Can you work these out from the model? Positions are in its coordinate system, mm. Face numbers are marked on the shaded views. A direction names the side the tool comes from. Give positions to 0.01 mm unless a question says otherwise; leave off trailing zeros. Write each loop counter-clockwise with the first axis right and the second up, starting at its lowest first coordinate (ties: lowest second). Pieces come first, ordered by that corner, then holes. Notation, with made-up numbers: (-34, -29.75) -> (-20, -29.75) arc R14 cw to (-20, -6.75) -> close; hole circle Ø7 at (64, 74). An arc over 180 degrees is marked (long way). One line per item, written item: value.
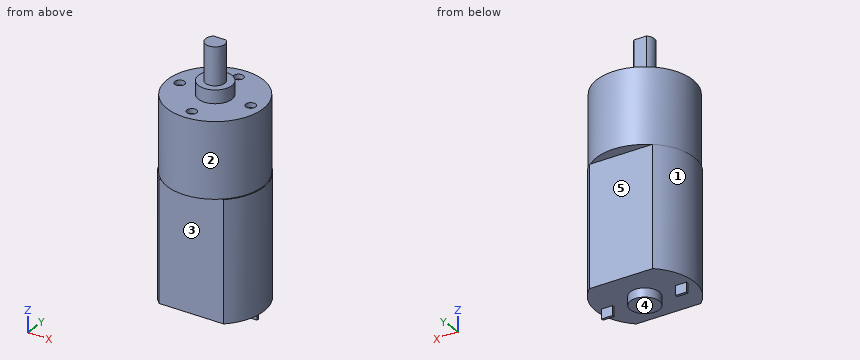
from build123d import *

# Parameters (mm, degrees)
SKETCH1_R                    = 10
GEARBOX_DEPTH                = 15.7
MOTOR_DEPTH                  = 25.1
SKETCH4_R                    = 3.5
OUTPUT_SHAFT_COLLAR_DEPTH    = 2.78
OUTPUT_SHAFT_DEPTH           = 7.87
SKETCH6_R                    = 3.02
BOSS_EXTRUDE11_DEPTH         = 1.86
SKETCH10_W                   = 2.36
SKETCH10_H                   = 0.5
BOSS_EXTRUDE13_DEPTH         = 2
M2_5X0_45_TAPPED_HOLE1_D     = 2.05
M2_5X0_45_TAPPED_HOLE1_DEPTH = 1
M2_5X0_45_TAPPED_HOLE1_TIP   = 0.615882135


with BuildPart() as part:
    # Sketch1 → GearBox (new body)
    with BuildSketch(Plane.XY):
        Circle(SKETCH1_R)
    extrude(amount=GEARBOX_DEPTH)

    # Sketch3 → Motor (add)
    with BuildSketch(Plane(origin=(0, 0, 0), x_dir=(-1, 0, 0), z_dir=(0, 0, -1))):
        with BuildLine():
            Line((-6.674371666, 7.65), (6.674371666, 7.65))
            ThreePointArc((6.674371666, 7.65), (10.2, 0.032634765), (6.818960021, -7.65))
            Line((6.818960021, -7.65), (-6.818960021, -7.65))
            ThreePointArc((-6.818960021, -7.65), (-10.2, 0.032634765), (-6.674371666, 7.65))
        make_face()
    extrude(amount=MOTOR_DEPTH)

    # Sketch4 → Output_Shaft_Collar (add)
    with BuildSketch(Plane.XY.offset(15.7)):
        Circle(SKETCH4_R)
    extrude(amount=OUTPUT_SHAFT_COLLAR_DEPTH)

    # Sketch5 → Output_Shaft (add)
    with BuildSketch(Plane.XY.offset(18.48)):
        with BuildLine():
            Line((-1.322875656, 1.5), (1.322875656, 1.5))
            ThreePointArc((1.322875656, 1.5), (0, -2), (-1.322875656, 1.5))
        make_face()
    extrude(amount=OUTPUT_SHAFT_DEPTH)

    # Sketch6 → Boss-Extrude11 (add)
    with BuildSketch(Plane(origin=(0, 0, -25.1), x_dir=(-1, 0, 0), z_dir=(0, 0, -1))):
        Circle(SKETCH6_R)
    extrude(amount=BOSS_EXTRUDE11_DEPTH)

    # Sketch10 → Boss-Extrude13 (add)
    with BuildSketch(Plane(origin=(0, 0, -25.1), x_dir=(-1, 0, 0), z_dir=(0, 0, -1))):
        with Locations((-7.82, 0)):
            Rectangle(SKETCH10_W, SKETCH10_H)
        with Locations((7.82, 0)):
            Rectangle(SKETCH10_W, SKETCH10_H)
    extrude(amount=BOSS_EXTRUDE13_DEPTH)

    # M2.5x0.45 Tapped Hole1
    with Locations(Plane.XY.offset(15.7)):
        with Locations((-7.5, 0), (7.5, 0), (0, 7.5), (0, -7.5)):
            Hole(M2_5X0_45_TAPPED_HOLE1_D / 2, depth=M2_5X0_45_TAPPED_HOLE1_DEPTH)
            with Locations((0, 0, -(M2_5X0_45_TAPPED_HOLE1_DEPTH + M2_5X0_45_TAPPED_HOLE1_TIP / 2))):  # 118° drill point
                Cone(0, M2_5X0_45_TAPPED_HOLE1_D / 2, M2_5X0_45_TAPPED_HOLE1_TIP, mode=Mode.SUBTRACT)


solid = part.part
1) I need wall thicknesses on L1, parallel to X at y = 0, z = 15.2 (3 decimals); L2, parallel to Y at x = -1.75, z = -25. Which ranges of each line are inside material? Lowest first, please.
Answer list:
L1: x = -10 to -8.525, -6.475 to 6.475, 8.525 to 10
L2: y = -7.65 to 7.65
2) If we section it at B-B (z = -1.5): Write out the boundary of the cut face in (x, y), and give its area (3 significant figures).
Answer list:
outline: (-6.82, -7.65) -> (6.82, -7.65) arc R10.2 ccw to (6.67, 7.65) -> (-6.67, 7.65) arc R10.2 ccw to start
area: 280 mm^2
3) If we section it at C-C (x = -5): Write out the boundary of the cut face in (y, z).
Answer list:
outline: (-8.66, 0) -> (-7.65, 0) -> (-7.65, -25.1) -> (7.65, -25.1) -> (7.65, 0) -> (8.66, 0) -> (8.66, 15.7) -> (-8.66, 15.7) -> close
4) If we section it at A-A (x = 4.5): Write out the boundary of the cut face in (y, z), and give its area (3 significant figures).
Answer list:
outline: (-8.93, 0) -> (-7.65, 0) -> (-7.65, -25.1) -> (7.65, -25.1) -> (7.65, 0) -> (8.93, 0) -> (8.93, 15.7) -> (-8.93, 15.7) -> close
area: 664 mm^2
5) For the marked faces 1, 2, 3, 4 and 5, which set-ups out of +Z, -Z, +X, -X, +Y, -Y let a thin tool reach every point of the face, with its end or its side?
Answer list:
face 1: +Z, -Z, -X
face 2: +Z
face 3: -Z, +X, -X, -Y
face 4: -Z, +Y, -Y
face 5: -Z, +X, -X, +Y
6) Will these pins go through, and if not, where does the flat tip stop? pin 1 (3 mm diameter, centred on x = 0.5, y = -5, fed in from -Z); pin 2 (2.5 mm diameter, centred on x = 0, y = 7.5, fed in from +Z); pin 3 (12 mm diameter, centred on x = -3.5, y = -7.5, fed in from -Z).
Answer list:
pin 1: stops at z = -25.1
pin 2: stops at z = 15.7
pin 3: stops at z = -26.96
